Could you check a few things on this model? Use its own coordinates, in mm. A direction names the side the tool comes from. Give positions to 0.01 mm unless a question says otherwise; leave off trailing zeros. Loops run counter-clockwise (first coordinate to the right, second up) from the corner with the lowest first, then second, coordinate; pieces in that order, holes last. Notation, with made-up numbers: M 64.25,63 L 123.25,63 A11 cw 123.25,74 Z; hole C -7,-13 d5. An arc over 180 degrees is marked long. Answer in a Markdown table with one row per item. Add a question column.
```python
from build123d import *

# Parameters (mm, degrees)
F1_R     = 3.4943107557
F1_R_2   = 3.0428811149
F2_DEPTH = 5
F1_R_3   = 4.5
F3_DEPTH = 5
F0_R     = 4.5
F0_R_2   = 2.5
F0_R_3   = 1.2499972105
F4_DEPTH = 1.5
F5_DEPTH = 5


with BuildPart() as f2:
    # F1 (on Top) → F2 (new body)
    with BuildSketch(Plane.XY):
        with Locations((0.0001326702, 0.0020665845)):
            Circle(F1_R)
        with Locations((-0.0001288142, 0.0001297904)):
            Circle(F1_R_2, mode=Mode.SUBTRACT)
    extrude(amount=F2_DEPTH)

    # F1 (on Top) → F3 (join)
    with BuildSketch(Plane.XY):
        with Locations((-0.0001288142, 0.0001297904)):
            Circle(F1_R_3)
        with Locations((0.0001326702, 0.0020665845)):
            Circle(F1_R, mode=Mode.SUBTRACT)
    extrude(amount=F3_DEPTH)

    # F0 (on Top) + F1 (on Top) → F4 (join)
    with BuildSketch(Plane.XY):
        with BuildLine():
            Line((2.4394025121, -12.0658558892), (4.2479218755, -4.2443155336))
            Line((4.2479218755, -4.2443155336), (12.0694627081, -2.4357959317))
            ThreePointArc((12.0694627081, -2.4357959317), (13.9939445399, 0.0026156227), (12.0586423193, 2.4324482394))
            Line((12.0586423193, 2.4324482394), (4.240708283, 4.2373605681))
            Line((4.240708283, 4.2373605681), (2.4321889196, 12.0589037848))
            ThreePointArc((2.4321889196, 12.0589037848), (-0.0037356104, 13.9965222261), (-2.4396601404, 12.0589037848))
            Line((-2.4396601404, 12.0589037848), (-4.2436064604, 4.240965457))
            Line((-4.2436064604, 4.240965457), (-12.0625067438, 2.4360531283))
            ThreePointArc((-12.0625067438, 2.4360531283), (-14.000128813, 0.0001285983), (-12.0625067438, -2.4357959317))
            Line((-12.0625067438, -2.4357959317), (-4.2409659113, -4.2443155336))
            Line((-4.2409659113, -4.2443155336), (-2.4324465479, -12.0658558892))
            ThreePointArc((-2.4324465479, -12.0658558892), (0.0034779821, -14.0034779629), (2.4394025121, -12.0658558892))
        make_face()
        with Locations((-0.0001288142, 0.0001297904)):
            Circle(F0_R, mode=Mode.SUBTRACT)
        with Locations((-0.0001288142, 0.0001297904)):
            Circle(F0_R)
        with Locations((-0.0001288142, 0.0001297904)):
            Circle(F0_R_2, mode=Mode.SUBTRACT)
        with Locations((-0.0001288142, 0.0001297904)):
            Circle(F0_R_2)
        with Locations((-0.0001288142, 0.0001297904)):
            Circle(F0_R_3, mode=Mode.SUBTRACT)
    with BuildSketch(Plane.XY):
        with Locations((0.0001326702, 0.0020665845)):
            Circle(F1_R)
        with Locations((-0.0001288142, 0.0001297904)):
            Circle(F1_R_2, mode=Mode.SUBTRACT)
    extrude(amount=F4_DEPTH)

    # F1 (on Top) → F5 (join)
    with BuildSketch(Plane.XY):
        with Locations((-0.0001288142, 0.0001297904)):
            Circle(F1_R_2)
        Polygon((2.5888910537, 0.6508482021), (2.3615180848, 0.4162336288), (2.6700632073, -0.0415643753), (2.3897163069, -0.2093383499), (2.5692487953, -0.7313942032), (2.2550279187, -0.8208914163), (2.2933322567, -1.3716230342), (1.9666683684, -1.3767441826), (1.861117768, -1.9186296846), (1.5442495959, -1.8390229053), (1.3020652759, -2.3351228771), (1.0165907184, -2.1762260286), (0.6542527165, -2.5927414983), (0.419636276, -2.3653667199), (-0.0381593369, -2.6739021736), (-0.2059394501, -2.3935590213), (-0.7279900472, -2.5731005304), (-0.8174879323, -2.2588772947), (-1.3682272049, -2.2971816047), (-1.3733483173, -1.9705116288), (-1.9152342451, -1.8649690028), (-1.8356267052, -1.5480978036), (-2.3317276079, -1.3059049719), (-2.1728300866, -1.0204375874), (-2.5893344069, -0.6580942182), (-2.3619698137, -0.4234796389), (-2.6705078515, 0.0343198084), (-2.3901622681, 0.2020929949), (-2.5696944667, 0.7241480054), (-2.2554814608, 0.813645364), (-2.2937858509, 1.36437773), (-1.9671157465, 1.3694988444), (-1.8615737238, 1.9113816752), (-1.5447023894, 1.8317824829), (-1.3025083802, 2.3278777401), (-1.0170415808, 2.1689805445), (-0.6546890428, 2.5854941996), (-0.4200746079, 2.3581213648), (0.037725635, 2.6666599388), (0.205490485, 2.3863142801), (0.7275579628, 2.5658560526), (0.8170392653, 2.2516321833), (1.3677844908, 2.2899363469), (1.3728972309, 1.9632657859), (1.9147806544, 1.8577236477), (1.8351731146, 1.5408524485), (2.3312740172, 1.2986596169), (2.1723769594, 1.0131930648), align=None, mode=Mode.SUBTRACT)
    extrude(amount=F5_DEPTH)


solid = f2.part
```
Item 1: For P1, Ø2, axis at x = -8, y = 6, coming from the +Z side, with a flat end and sliding along its axis, tell me the tip position at first contact or that it passes through.
Item 2: For faces 1 (the face through (-3.33, 8.2, 0.74)), 2 (the face through (2.08, -3.99, 3.23)), which set-ups out of +Z, -Z, +X, -X, +Y, -Y let a thin tool reach every point of the face, with its end or its side?
Item 3: If we mould it in two halves opening along Y, with no side actions, what happens to faces 3 (the face through (3, 0, 0)), 4 (the face through (3.33, -8.21, 0.74)), 5 (the face through (-1, -1, 1.5)), 6 (the face through (0.672, 1.054, 0.74))? For each: +Y half, -Y half, draft (parallel to the pull), parting line (faces both ways), or undercut.
Item 4: Suppose I cut it at A-A (z = 0.8). List the corners of the cut face in (x, y) for me, then the cut area to 3 significant figures.
Item 5: Suppose I cut it at B-B (y = -3.25). List the corners of the cut face in (x, z) for me.
Item 6: Suppose I cut it at D-D (y = -11.5). List the corners of the cut face in (x, z) for me.
Item 7: I need wall thicknesses on L1, parallel to Z at x = 8.75, y = -1; L2, parallel to X at y = 0.25, z = 2.1; L3, parallel to Y at x = 12.25, z = 0.3. Which ranges of each line are inside material? Lowest first, please.
Item 8: Suppose I cut it at C-C (x = -5.5). List the corners of the cut face in (y, z) for me, then the cut area to 3 significant figures.
Values found:
| question | item | result |
|---|---|---|
| 1 | P1 | through |
| 2 | face 1 | +Z, -Z, -X, +Y |
| 2 | face 2 | +Z |
| 3 | face 3 | draft |
| 3 | face 4 | -Y half |
| 3 | face 5 | undercut |
| 3 | face 6 | undercut |
| 4 | outline | M -12.06,-2.44 L -4.24,-4.24 L -2.43,-12.07 A2.5 ccw 2.44,-12.07 L 4.25,-4.24 L 12.07,-2.44 A2.5 ccw 12.06,2.43 L 4.24,4.24 L 2.43,12.06 A2.5 ccw -2.44,12.06 L -4.24,4.24 L -12.06,2.44 A2.5 ccw Z; hole C 0,0 d2.5 |
| 4 | area | 304 mm² |
| 5 | outline | M -8.54,0 L 8.55,0 L 8.55,1.5 L 3.11,1.5 L 3.11,5 L -3.11,5 L -3.11,1.5 L -8.54,1.5 Z |
| 6 | outline | M -2.56,0 L 2.57,0 L 2.57,1.5 L -2.56,1.5 Z |
| 7 | L1 | 0 to 1.5 |
| 7 | L2 | -4.49 to -2.41, 2.47 to 4.49 |
| 7 | L3 | -2.39 to 2.38 |
| 8 | outline | M -3.95,0 L 3.95,0 L 3.95,1.5 L -3.95,1.5 Z |
| 8 | area | 11.9 mm² |
